Geometry: final body of the model. Coordinates: model frame, mm. Face numbers are marked on the shaded views. A direction names the side the tool comes from. Round coordinates to 2 decimals unless told otherwise and drop trailing zeros. Loops run counter-clockwise (first coordinate to the right, second up) from the corner with the lowest first, then second, coordinate; pieces in that order, holes last. Notation, with made-up numbers: (27, 82) - (81, 82) arc R14 cw to (81, 92) - close; hole circle Ø6 at (82, -14). An arc over 180 degrees is marked (long way). Write item = value, one per line. Start each with the question number.
Item 1: Section A-A (y = -33). Return loops of the section in (x, z) (3 decimals).
Item 2: First-contact query: pin 1 (1 mm diameter, centred on y = -36.5, z = 18, fed in from -X); pin 2 (4 mm diameter, centred on x = 20, y = -37, fed in from -Z); pin 3 (2.5 mm diameter, centred on x = 32.14, y = -36.97, fed in from +Z); pin 4 (1.1 mm diameter, centred on y = -28.5, z = 7, fed in from -X). Flat tips, straight axial feed; report the tip coordinate or a pass-through.
Item 3: Section B-B (x = 19). Return loops of the section in (y, z), plus the area to 3 significant figures.
Item 4: Draft query along X for the marked faces 4, 5 and 6. Return one class per face: pulls with the +X half, pulls with the -X half, needs draft (parallel to the pull), parting line crosses it, or undercut.
Item 5: Access query for the marked faces 1, 2 and 3. Directions: +Z, -Z, +X, -X, +Y, -Y. A direction counts if a zero-diameter tool reaches every point of the face in a straight line with its end or side. Return the directions, or none.
Item 6: Line query: line 1 (Y direction, x = 28.2, z = 20.3); line 2 (X direction, y = -39.75, z = 19.25); line 3 (X direction, y = -33.5, z = 18.5). Output: solid intervals per line, ascending. Write a range as from..to.
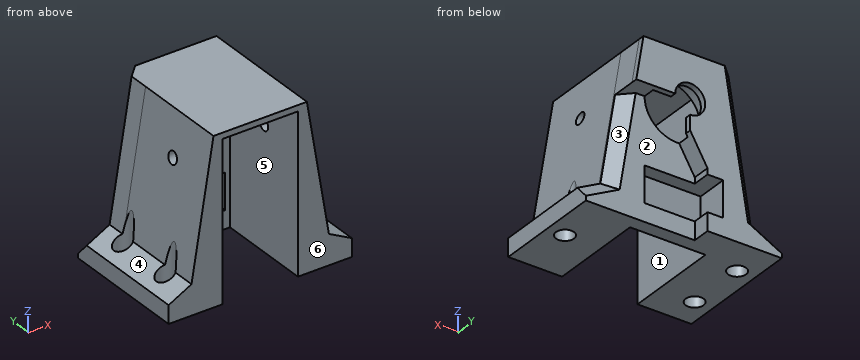
Autodesk Inventor part; units mm, degrees
ref_plane "YZ Plane" through (0, 0, 0) normal (1, 0, 0) x (0, 1, 0)
ref_plane "XZ Plane" through (0, 0, 0) normal (0, 1, 0) x (-1, 0, 0)
ref_plane "XY Plane" through (0, 0, 0) normal (0, 0, 1) x (1, 0, 0)
ref_plane "Work Plane1" through (14.3392, -46.1241, 0) normal (0, -1, 0) x (-1, 0, 0)
sketch "Sketch1" plane through (14.3392, -46.1241, 0) normal (0, -1, 0) x (-1, 0, 0)
  line L0 (-22.1702, 0) -> (47.1015, 0)
  line L1 (0.3, -25.8) -> (-11.3, -25.8) construction
  line L2 (-5.5, -25.8) -> (-5.5, 0) construction
  line L3 (0.8, 0) -> (0.8, -26.3)
  line L4 (0.8, -26.3) -> (-11.8, -26.3)
  line L5 (-11.8, -26.3) -> (-11.8, 0)
  line L6 (6.8, 0) -> (2.3, -27.3)
  line L7 (2.3, -27.3) -> (-13.3, -27.3)
  line L8 (-13.3, -27.3) -> (-17.8, 0)
  line L9 (5.9758, -5) -> (9.8, -3)
  line L10 (9.8, -3) -> (9.8, 0)
  line L11 (-16.9758, -5) -> (-20.8, -3)
  line L12 (-20.8, -3) -> (-20.8, 0)
  line L13 (5.9758, -5) -> (-16.9758, -5) construction
  line L14 (9.8, -3) -> (-20.8, -3) construction
  point P0 (14.3392, 0)
  dimension "d0" = 1
  dimension "d1" = 0.5
  dimension "d2" = 0.5
  dimension "d3" = 1.5
  dimension "d4" = 6
  dimension "d24" = 3
  dimension "d25" = 2
  dimension "d26" = 3
  dimension "d27" = 3
extrude "ext_maincage" add sketch "Sketch1" against normal blind 16 contours L0 L8 L11 L12 | L0 L5 L4 L3 L6 L7 L8 | L0 L10 L9 L6
sketch "Sketch2" plane through (14.3392, -30.1241, 0) normal (0, 1, 0) x (1, 0, 0)
  line L0 (-0.8, -26.3) -> (-0.8, 0)
  line L1 (-2.3, -27.3) -> (13.3, -27.3)
  line L2 (11.8, 0) -> (11.8, -26.3)
  line L3 (11.8, -26.3) -> (-0.8, -26.3)
  circle A0 centre (5.5, -20) radius 5.5
  circle A1 centre (5.5, -20) radius 7.3
  line L4 (-0.8, 0) -> (-0.8, -16.3122)
  line L5 (-0.8, -23.6878) -> (-0.8, -26.3)
  line L6 (-0.8, -26.3) -> (1.8122, -26.3)
  line L7 (9.1878, -26.3) -> (11.8, -26.3)
  line L8 (11.8, -23.6878) -> (11.8, -26.3)
  line L9 (-0.8, 0) -> (11.8, 0)
  line L10 (11.8, 0) -> (11.8, -16.3122)
  line L11 (-0.8, -16.3122) -> (-0.8, 0)
  line L12 (-0.8, 0) -> (-9.8, 0)
  line L13 (-9.8, 0) -> (-9.8, -3)
  line L14 (-9.8, -3) -> (-5.9758, -5)
  line L15 (-5.9758, -5) -> (-2.3, -27.3)
  line L16 (-2.3, -27.3) -> (13.3, -27.3)
  line L17 (13.3, -27.3) -> (16.9758, -5)
  line L18 (16.9758, -5) -> (20.8, -3)
  line L19 (20.8, -3) -> (20.8, 0)
  line L20 (20.8, 0) -> (11.8, 0)
  line L21 (11.8, 0) -> (11.8, -26.3)
  line L22 (11.8, -26.3) -> (-0.8, -26.3)
  line L23 (-0.8, -26.3) -> (-0.8, 0)
  point P0 (-6.8, 0)
  point P1 (17.8, 0)
  point P2 (-14.3392, 0)
  point P3 (3.5163, -12.9747)
  dimension "d7" = 11
extrude "ext_backhousing" add sketch "Sketch2" along normal blind 4.3
sketch "Sketch3" plane through (14.3392, -25.8241, 0) normal (0, 1, 0) x (1, 0, 0)
  line L0 (17.8, 0) -> (-6.8, 0)
  line L1 (-6.8, 0) -> (-2.3, -27.3)
  line L2 (-2.3, -27.3) -> (13.3, -27.3)
  line L3 (13.3, -27.3) -> (17.8, 0)
  circle A0 centre (5.5, -20) radius 2.5
  circle A1 centre (5.5, -20) radius 5.5
  line L4 (20.8, 0) -> (-9.8, 0)
  line L5 (-9.8, 0) -> (-9.8, -3)
  line L6 (-9.8, -3) -> (-5.9758, -5)
  line L7 (-5.9758, -5) -> (-2.3, -27.3)
  line L8 (-2.3, -27.3) -> (13.3, -27.3)
  line L9 (13.3, -27.3) -> (16.9758, -5)
  line L10 (16.9758, -5) -> (20.8, -3)
  line L11 (20.8, -3) -> (20.8, 0)
  point P0 (-0.8, 0)
  point P1 (-14.3392, 0)
  dimension "d10" = 5
extrude "ext_backcover" add sketch "Sketch3" along normal blind 1 contours L3 L2 L1 L0 | L4 L11 L10 L3 | L1 L6 L5 L4 | A1
sketch "Sketch4" plane through (14.3392, -24.8241, 0) normal (0, 1, 0) x (1, 0, 0)
  circle A0 centre (5.5, -20) radius 2.5
  line L0 (5.5, 0) -> (5.5, -17.5)
  line L1 (5.5, -15) -> (2.6132, -10)
  line L2 (2.6132, -10) -> (2.6132, 0)
  line L3 (20.8, 0) -> (-9.8, 0)
  line L4 (13.3, -27.3) -> (16.9758, -5)
  line L5 (20.8, -3) -> (20.8, 0)
  line L6 (8, -20) -> (14.5033, -20)
  line L7 (-2.3, -27.3) -> (13.3, -27.3)
  line L8 (16.9758, -5) -> (20.8, -3)
  circle A1 centre (5.5, -20) radius 2.5
  line L9 (14.5643, -19.6299) -> (16.9758, -5)
  line L10 (16.9758, -5) -> (20.8, -3)
  line L11 (20.8, -3) -> (20.8, 0)
  line L12 (20.8, 0) -> (5.5, 0)
  point P0 (-14.3392, 0)
  dimension "d22" = 30
  dimension "d23" = 10
  dimension "d28" = 5
extrude "ext_cut_backcutway" cut sketch "Sketch4" against normal blind 3 contours A0 L0 L3 L5 L8 L4 L6 | L1 L2 L3 L0
chamfer "Chamfer3" distance 2 angle 45 4 edges at (30.0788, -27.8241, 12.5) (33.2272, -27.8241, 4) (6.4513, -24.8241, 4) (10.2013, -24.8241, 16.15)
ref_plane "back_plane" through (14.3392, -24.8241, 0) normal (0, 1, 0) x (1, 0, 0)
sketch "Sketch5" plane through (14.3392, -24.8241, 0) normal (0, 1, 0) x (1, 0, 0)
  line L0 (-0.273, -27.3) -> (13.3, -27.3)
  line L1 (2.6132, 0) -> (20.8, 0)
  line L2 (11, -9) -> (11, -3)
  line L3 (11, -3) -> (0, -3)
  line L4 (0, -3) -> (0, -9)
  line L5 (0, -9) -> (11, -9)
  line L6 (11, -9) -> (0, -3) construction
  line L7 (11, -3) -> (0, -9) construction
  arc A0 (5.5, -17.5) -> (8, -20) centre (5.5, -20) ccw
  line L8 (5.5, -20) -> (5.5, -3) construction
  point P0 (-14.3392, 0)
  point P1 (5.5, -6)
  point P2 (5.5, -6)
  dimension "d33" = 6
  dimension "d34" = 11
  dimension "d37" = 3
extrude "Extrusion5" cut sketch "Sketch5" against normal through all
sketch "Sketch6" plane through (0, 0, 0) normal (0, 0, 1) x (1, 0, 0)
  line L0 (35.1392, -46.1241) -> (35.1392, -27.8241)
  circle A0 centre (32.1392, -36.9741) radius 1.5
  line L1 (33.6392, -36.9741) -> (35.1392, -36.9741)
  line L2 (32.1392, -36.9741) -> (33.6392, -36.9741) construction
  line L3 (4.5392, -46.1241) -> (4.5392, -26.8241)
  line L4 (4.5392, -46.1241) -> (4.5392, -24.8241)
  circle A1 centre (7.5392, -31.1241) radius 1.5
  circle A2 centre (7.5392, -41.1241) radius 1.5
  line L5 (7.5392, -31.1241) -> (7.5392, -41.1241) construction
  line L6 (7.5392, -41.1241) -> (6.0392, -41.1241) construction
  line L7 (7.5392, -31.1241) -> (6.0392, -31.1241) construction
  line L8 (4.5392, -31.1241) -> (6.0392, -31.1241)
  line L9 (4.5392, -41.1241) -> (6.0392, -41.1241)
  line L10 (35.1392, -46.1241) -> (35.1392, -29.8241)
  point P0 (0, 0)
  dimension "d38" = 3
  dimension "d40" = 1.5
  dimension "d43" = 10
  dimension "d44" = 5
extrude "Extrusion6" cut sketch "Sketch6" along normal through all
sketch "Sketch7" plane through (26.1392, -46.1241, 0) normal (-1, 0, 0) x (0, 0, 1)
  line L0 (26.3, 0) -> (26.3, 16)
  line L1 (0, 0) -> (0, 16)
  line L2 (26.3, 8) -> (0, 8) construction
  circle A0 centre (20.3, 8) radius 1
  point P0 (0, 46.1241)
  dimension "d47" = 2
  dimension "d48" = 6
extrude "Extrusion7" cut sketch "Sketch7" along normal through all both and the other way through all
equation "\"d7\" = linact_bearing_diameter"
equation "\"d8\" = linact_bearing_thickness"
equation "\"d38\" = screw_m3_bore_selfthreading"
equation "\"d47\" = screw_m2_bore_selfthreading"
properties part number "servo_clamp"
Taken from the geometry:
q1.outline = (4.539, 0) - (13.539, 0) - (13.539, 26.3) - (26.139, 26.3) - (26.139, 0) - (35.139, 0) - (35.139, 3) - (31.315, 5) - (27.639, 27.3) - (12.039, 27.3) - (8.363, 5) - (4.539, 3) - close
q2.pin_1 = 10.42
q2.pin_2 = 26.3
q2.pin_3 = through
q2.pin_4 = 8.6
q3.outline = (-46.12, 26.3) - (-30.12, 26.3) - (-30.12, 25.44) - (-25.82, 25.44) - (-25.82, 22.35) - (-24.82, 22.35) - (-24.82, 27.3) - (-46.12, 27.3) - close; (-30.12, 0) - (-27.82, 0) - (-27.82, 3) - (-30.12, 3) - close; (-30.12, 9) - (-27.82, 9) - (-27.82, 13.55) - (-24.82, 13.55) - (-24.82, 17.65) - (-25.82, 17.65) - (-25.82, 14.56) - (-30.12, 14.56) - close
q3.area = 54.8 mm^2
q4.face_4 = pulls with the -X half
q4.face_5 = undercut
q4.face_6 = needs draft
q5.face_1 = -Z, -Y
q5.face_2 = -Z, +X, +Y
q5.face_3 = +X, +Y
q6.line_1 = -46.12..-39.12, -37.12..-24.82
q6.line_2 = 10.71..13.54, 26.14..28.97
q6.line_3 = 10.59..13.54, 26.14..29.09
